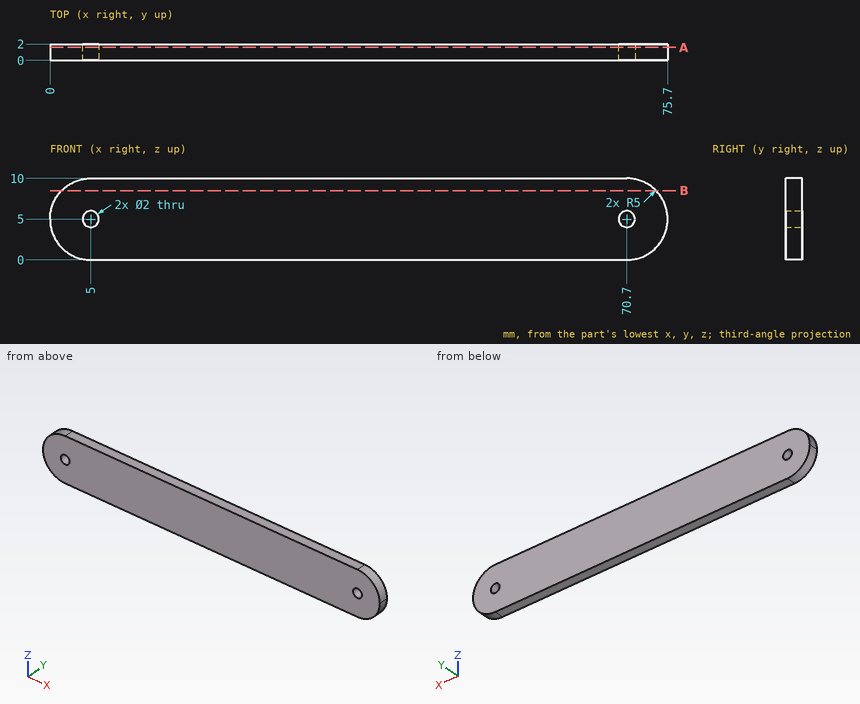
Answer from the drawing. Dimensions are ordinates in mm from the lowest x, y and z of the part. Round coordinates to 2 decimals unless told otherwise and drop trailing zeros. Order: outer loops, then holes, each group sorted by start corner. A loop starts at its lowest first (then second) coordinate and runs counter-clockwise, first axis right, second up.
1) The part is cut by section A-A on y = 1.6. Give the number of separate pieces and of enclosed holes in the cut face, plus the area to 3 significant figures.
2) A flat-ended cylindrical pin translates along its axis: pin 1 (1 mm diameter, centred on y = 0.5, z = 1.5, fed in from -X). Find the tip coordinate at first contact, or state that the pin passes through.
3) The part is cut by section B-B on z = 8.5. Write down the section's boundary in (x, y).
4) Straight lines are drawn through the part: L1, parallel to Z at x = 5, y = 1.3; L2, parallel to X at y = 1.95, z = 6.25; L3, parallel to X at y = 1.2, z = 1.75. For each, find the intervals that lie inside material, in ascending order.
Resolved:
1. separate pieces: 1
1. enclosed holes: 2
1. area: 729 mm2
2. pin 1: stops at x = 1
3. outline: (1.43, 0) - (74.27, 0) - (74.27, 2) - (1.43, 2) - close
4. L1: z = 0 to 4, 6 to 10
4. L2: x = 0.16 to 75.54
4. L3: x = 1.2 to 74.5
